Autodesk Inventor part; units mm, degrees
ref_plane "YZ Plane" through (0, 0, 0) normal (1, 0, 0) x (0, 1, 0)
ref_plane "XZ Plane" through (0, 0, 0) normal (0, 1, 0) x (-1, 0, 0)
ref_plane "XY Plane" through (0, 0, 0) normal (0, 0, 1) x (1, 0, 0)
ref_plane "РабПлоскость1" through (8.6347, 23.8825, 435.6127) normal (0, 0, 1) x (0, -1, 0)
sketch "Эскиз1" plane through (8.6347, 23.8825, 435.6127) normal (0, 0, 1) x (0, -1, 0)
  line L0 (11.5, 6) -> (11.5, -6)
  line L1 (15, -6) -> (11.5, -6)
  arc A0 (15, -6) -> (16, -5) centre (15, -5) ccw
  line L2 (16, -1.25) -> (16, -5)
  line L3 (14, -1.25) -> (16, -1.25)
  arc A1 (12.8, -0.05) -> (14, -1.25) centre (14, -0.05) ccw
  line L4 (12.8, 0.05) -> (12.8, -0.05)
  arc A2 (14, 1.25) -> (12.8, 0.05) centre (14, 0.05) ccw
  line L5 (16, 1.25) -> (14, 1.25)
  line L6 (16, 5) -> (16, 1.25)
  arc A3 (16, 5) -> (15, 6) centre (15, 5) ccw
  line L7 (11.5, 6) -> (15, 6)
  circle A4 centre (13.75, 3.5) radius 1.25
  circle A5 centre (13.75, -3.5) radius 1.25
  line L8 (11.5, 6) -> (17.129, 6)
  line L9 (17.129, 6) -> (17.129, -46.099)
  line L10 (17.129, -46.099) -> (11.5, -46.099)
  line L11 (11.5, -46.099) -> (11.5, 6)
  point P0 (23.8825, -8.6347)
  point P1 (15, 6)
extrude "Выдавливание1" add sketch "Эскиз1" along normal blind 6
sketch "Эскиз2" plane through (-37.4643, 12.3825, 435.6127) normal (0, 1, 0) x (1, 0, 0)
  circle A0 centre (12.4913, -3) radius 1.5
  line L0 (52.099, -6) -> (0, -6)
  line L1 (0, 0) -> (52.099, 0)
  line L2 (5.2913, 0) -> (19.5913, 0)
  line L3 (19.5913, 0) -> (19.5913, -6)
  line L4 (19.5913, -6) -> (5.2913, -6)
  line L5 (5.2913, -6) -> (5.2913, 0)
  point P0 (37.4643, 435.6127)
  point P1 (5.2913, -3)
  point P2 (19.5913, 0)
  dimension "d2" = 3
  dimension "d3" = 3
  dimension "d4" = 7.2
  dimension "d5" = 7.1
extrude "Выдавливание2" cut sketch "Эскиз2" against normal blind 2
extrude "Выдавливание3" cut sketch "Эскиз2" against normal through all contours A0
properties part number "крепеж тсрт"
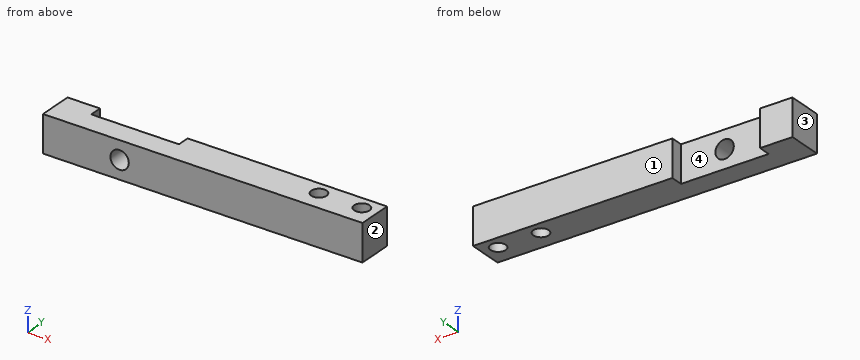
The listing builds one solid part. Answer for the finished solid, in the listing's coordinates (mm). Face numbers are marked on the shaded views. Round coordinates to 2 decimals unless told otherwise and drop trailing zeros. Order: outer loops, then holes, each group sorted by start corner. A loop starts at its lowest first (then second) coordinate and runs counter-clockwise, first axis right, second up. Notation, with made-up numbers: (26, 46.25) - (31, 46.25) arc R10 ccw to (31, 52.25) - close; hole circle Ø9 at (-27, -30.75). An arc over 180 degrees is marked (long way). Put each result on its own line as item: value. Start each with the question number.
(1) Determine the mould class of the marked faces 1, 2, 3 and 4 for opening direction X: released by +X, released by -X, zero draft, split by the parting line, or undercut.
(2) Straight lines are drawn through the part: probe 1 along X at (y, z) = (10.05, 436.9); probe 2 along X at (y, z) = (10.9, 440.55); probe 3 along X at (y, z) = (10.6, 435.9). For each, find the intervals that lie inside material, in ascending order. Write a range as from..to.
(3) Find section D-D (z = 437.6). Give the vertices of the cut face in (x, y), plus the area to 3 significant figures.
(4) Given P1, Ø3, axis at x = 5.13, y = 10.13, coming from the -Z side; P2, Ø2, axis at x = 12.13, y = 10.13, coming from the -Z side, each flat-ended and moving along its own axis, determine where each tip first touches the part or whether it passes through.
(5) Find section B-B (y = 9.55). Give the vertices of the cut face in (x, z), plus the area to 3 significant figures.
(6) Find section C-C (x = -25). Give the vertices of the cut face in (y, z), plus the area to 3 significant figures.
(7) Find section A-A (z = 439.5). Give the vertices of the cut face in (x, y).
Reply:
1. face 1: zero draft
1. face 2: released by +X
1. face 3: released by -X
1. face 4: undercut
2. probe 1: -37.46..3.89, 6.38..10.89, 13.38..14.63
2. probe 2: -37.46..-32.17, -17.87..4.15, 6.12..11.15, 13.12..14.63
2. probe 3: -37.46..-32.17, -17.87..3.98, 6.29..10.98, 13.29..14.63
3. outline: (-37.46, 6.75) - (-26.08, 6.75) - (-26.08, 10.38) - (-32.17, 10.38) - (-32.17, 12.38) - (-37.46, 12.38) - close; (-23.87, 6.75) - (14.63, 6.75) - (14.63, 12.38) - (-17.87, 12.38) - (-17.87, 10.38) - (-23.87, 10.38) - close; hole circle Ø2.5 at (5.13, 10.13); hole circle Ø2.5 at (12.13, 10.13)
3. area: 247 mm^2
4. P1: z = 435.61
4. P2: through
5. outline: (-37.46, 435.61) - (4.03, 435.61) - (4.03, 441.61) - (-37.46, 441.61) - close; (6.24, 435.61) - (11.03, 435.61) - (11.03, 441.61) - (6.24, 441.61) - close; (13.24, 435.61) - (14.63, 435.61) - (14.63, 441.61) - (13.24, 441.61) - close; hole circle Ø3 at (-24.97, 438.61)
5. area: 279 mm^2
6. outline: (6.75, 435.61) - (10.38, 435.61) - (10.38, 437.11) - (6.75, 437.11) - close; (6.75, 440.11) - (10.38, 440.11) - (10.38, 441.61) - (6.75, 441.61) - close
6. area: 10.9 mm^2
7. outline: (-37.46, 6.75) - (-26.18, 6.75) - (-26.18, 10.38) - (-32.17, 10.38) - (-32.17, 12.38) - (-37.46, 12.38) - close; (-23.76, 6.75) - (14.63, 6.75) - (14.63, 12.38) - (-17.87, 12.38) - (-17.87, 10.38) - (-23.76, 10.38) - close; hole circle Ø2.5 at (5.13, 10.13); hole circle Ø2.5 at (12.13, 10.13)
